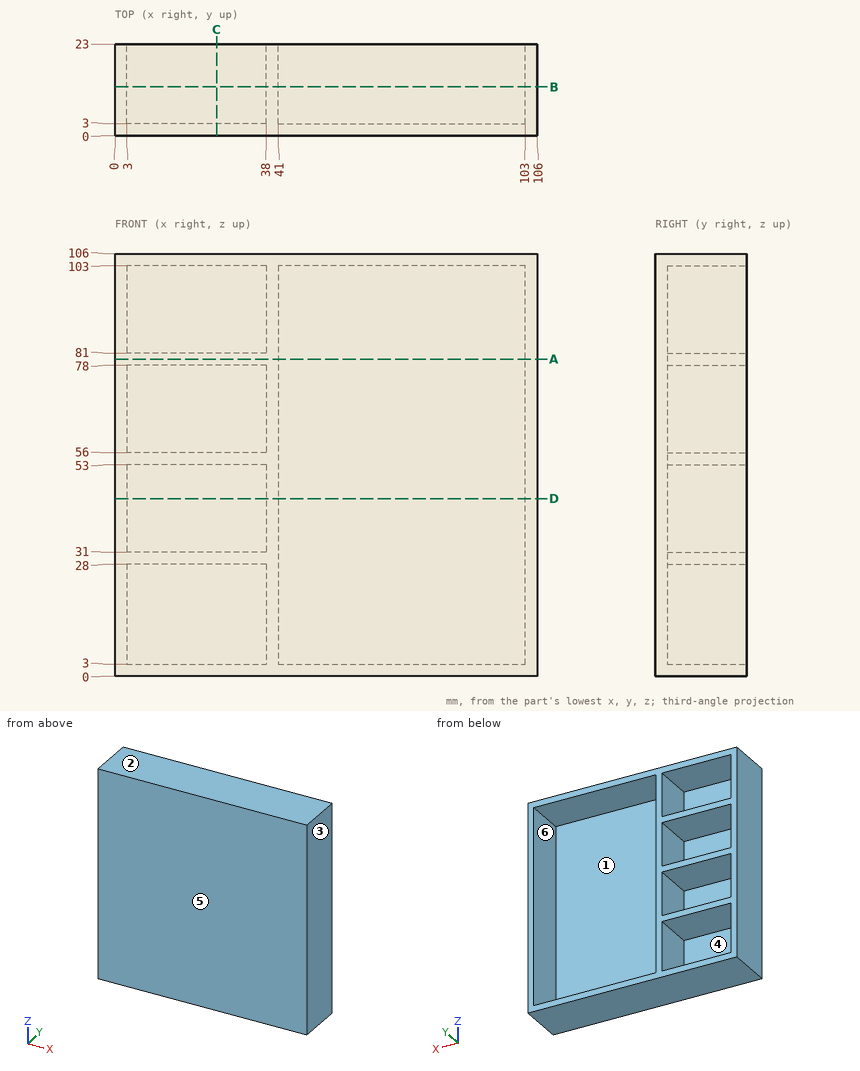
Geometry: see drawing. Coordinates: mm, zero at the bounding-box minimum. A direction names the side the tool comes from. Coordinates: 2 decimals unless noted, no trailing zeros. Loops run counter-clockwise (first coordinate to the right, second up) from the corner with the lowest first, then second, coordinate; pieces in that order, holes last. Notation, with made-up numbers: (50, 86.5) -> (79, 86.5) arc R19 cw to (79, 116.5) -> close; hole circle Ø10 at (32, -36.75). An arc over 180 degrees is marked (long way). Write item = value, one per line. Start each with the question number.
Item 1: First-contact query: P1, Ø1.5, axis at x = 26, y = 13.5, coming from the -Z side; P2, Ø1, axis at x = 82, z = 77, coming from the +Y side. Flat tips, straight axial feed; report the tip coordinate or a pass-through.
Item 2: Mould query, pull axis X, two halves, no side actions, for the marked faces 1, 2, 3 and 4. Classes: pulls with the +X half, pulls with the -X half, needs draft (parallel to the pull), parting line crosses it, or undercut.
Item 3: Cut plane B-B, the plane y = 12.25. Return loops of the section in (x, z).
Item 4: Cut plane D-D, the plane z = 44.5. Return loops of the section in (x, y), plus the area to 3 significant figures.
Item 5: Cut plane C-C, the plane x = 25.5. Return loops of the section in (y, z).
Item 6: Material intervals for line 1 (X direction, y = 8, z = 25); line 2 (Z direction, x = 6.5, y = 21.5); line 3 (Z direction, x = 69, y = 4), sorted ascending.
Item 7: Cut plane A-A, the plane z = 79.5. Return loops of the section in (x, y), plus the area to 3 significant figures.
Item 8: Reachability of the marked faces 5 and 6 from +Z, -Z, +X, -X, +Y, -Y: full face, straight path, thin tool, end or side. Return the list, or none.
Ans:
q1.P1 = 0
q1.P2 = 3
q2.face_1 = undercut
q2.face_2 = needs draft
q2.face_3 = pulls with the +X half
q2.face_4 = undercut
q3.outline = (0, 0) -> (106, 0) -> (106, 106) -> (0, 106) -> close; hole (3, 3) -> (38, 3) -> (38, 28) -> (3, 28) -> close; hole (3, 31) -> (38, 31) -> (38, 53) -> (3, 53) -> close; hole (3, 56) -> (38, 56) -> (38, 78) -> (3, 78) -> close; hole (3, 81) -> (38, 81) -> (38, 103) -> (3, 103) -> close; hole (41, 3) -> (103, 3) -> (103, 103) -> (41, 103) -> close
q4.outline = (0, 0) -> (106, 0) -> (106, 23) -> (103, 23) -> (103, 3) -> (41, 3) -> (41, 23) -> (38, 23) -> (38, 3) -> (3, 3) -> (3, 23) -> (0, 23) -> close
q4.area = 498 mm²
q5.outline = (0, 0) -> (23, 0) -> (23, 3) -> (3, 3) -> (3, 28) -> (23, 28) -> (23, 31) -> (3, 31) -> (3, 53) -> (23, 53) -> (23, 56) -> (3, 56) -> (3, 78) -> (23, 78) -> (23, 81) -> (3, 81) -> (3, 103) -> (23, 103) -> (23, 106) -> (0, 106) -> close
q6.line_1 = 0 to 3, 38 to 41, 103 to 106
q6.line_2 = 0 to 3, 28 to 31, 53 to 56, 78 to 81, 103 to 106
q6.line_3 = 0 to 3, 103 to 106
q7.outline = (0, 0) -> (106, 0) -> (106, 23) -> (103, 23) -> (103, 3) -> (41, 3) -> (41, 23) -> (0, 23) -> close
q7.area = 1,200 mm²
q8.face_5 = +Z, -Z, +X, -X, -Y
q8.face_6 = +Y
